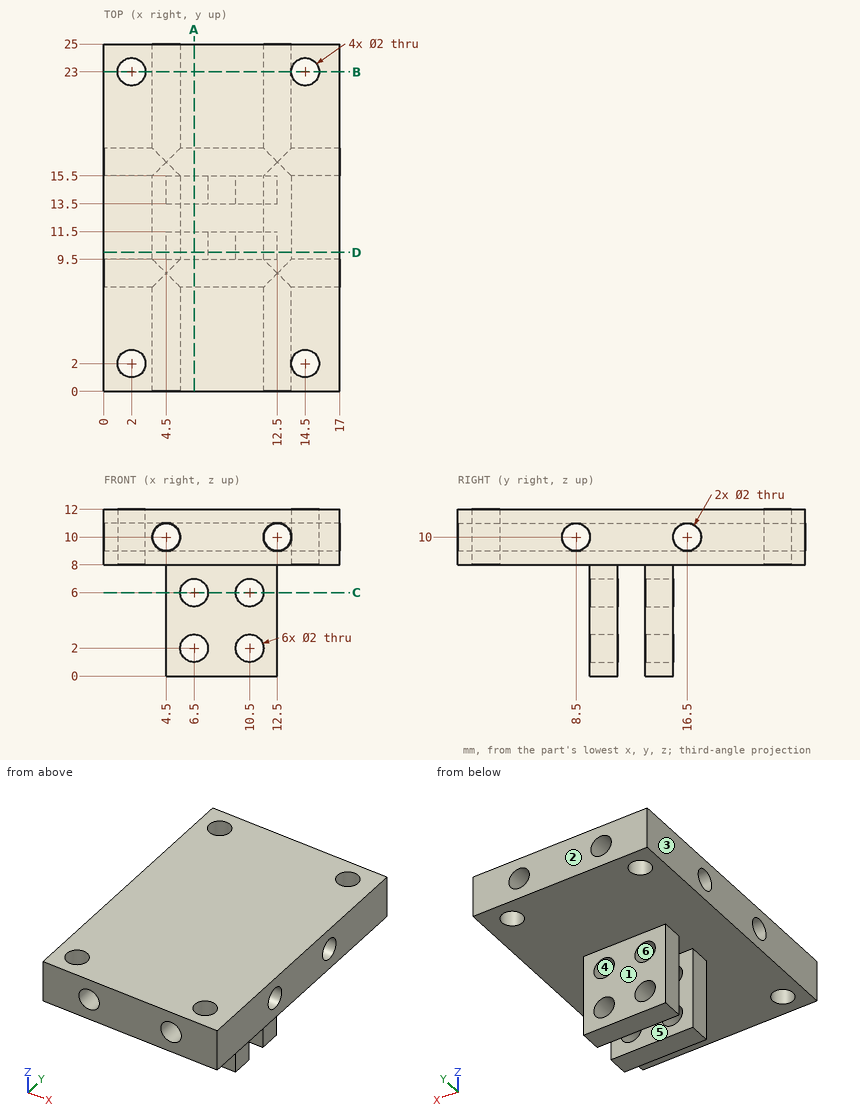
Could you check a few things on this drawing? It's one solid part, dimensions in mm from its lowest x, y, z. A direction names the side the tool comes from. Coordinates: 2 decimals unless noted, no trailing zeros. Order: outer loops, then holes, each group sorted by start corner. A loop starts at its lowest first (then second) coordinate and runs counter-clockwise, first axis right, second up. Notation, with made-up numbers: M 79,49 L 130,49 A30 ccw 130,84 Z; hole C 12.5,29 d2. An arc over 180 degrees is marked long. Answer as a JSON object with one key per item and string values. Group by question number.
(1) Which directions (+Z, -Z, +X, -X, +Y, -Y) give clear straight access to the entire face, cutting with the end or side of a thin tool? Please do the marked faces 1 and 2.
(2) For pin 1 (2.5 mm diameter, centred on x = 10, z = 4.5, fed in from +Y); pin 2 (1.2 mm diameter, centred on x = 12.5, z = 10, fed in from +Y); pin 3 (2 mm diameter, centred on y = 14.5, z = 5, fed in from +X); pin 4 (3 mm diameter, centred on x = 4, y = 20.5, fed in from -Z), each with a flat end and sliding along its axis, tell me the tip position at first contact or that it passes through.
(3) I need wall thicknesses on probe 1 along Z at (x, y) = (10.5, 14.1); probe 2 along X at (y, z) = (11.5, 10); probe 3 along Y at (x, z) = (10.25, 10). Which ranges of each line are inside material? Lowest first, please.
(4) Suppose I cut it at C-C, the plane z = 6. Please give me the cut outline in (x, y), then the cut area to 3 significant figures.
(5) Suppose I cut it at B-B, the plane y = 23. Please give me the cut outline in (x, z).
(6) If we mould it in two halves opening along X, with no side actions, what happens to the marked faces 3, 4, 5 and 6? For each: released by +X, released by -X, zero draft, split by the parting line, or undercut.
(7) Suppose I cut it at D-D, the plane y = 10. Please give me the cut outline in (x, z), then the cut area to 3 significant figures.
(8) Suppose I cut it at A-A, the plane x = 6.5. State how many separate pieces and enclosed holes the cut face has, then the cut area to 3 significant figures.
Values found:
{
 "1": {"face 1": "-Z, +X, -X, +Y", "face 2": "+Z, -Z, +X, -X, +Y"},
 "2": {"pin 1": "stops at y = 15.5", "pin 2": "passes through", "pin 3": "stops at x = 12.5", "pin 4": "stops at z = 8"},
 "3": {"probe 1": "z = 0 to 1, 3 to 5, 7 to 12", "probe 2": "x = 0 to 3.5, 5.5 to 11.5, 13.5 to 17", "probe 3": "y = 0 to 7.5, 9.5 to 15.5, 17.5 to 25"},
 "4": {"outline": "M 4.5,9.5 L 5.5,9.5 L 5.5,11.5 L 4.5,11.5 Z; M 4.5,13.5 L 5.5,13.5 L 5.5,15.5 L 4.5,15.5 Z; M 7.5,9.5 L 9.5,9.5 L 9.5,11.5 L 7.5,11.5 Z; M 7.5,13.5 L 9.5,13.5 L 9.5,15.5 L 7.5,15.5 Z; M 11.5,9.5 L 12.5,9.5 L 12.5,11.5 L 11.5,11.5 Z; M 11.5,13.5 L 12.5,13.5 L 12.5,15.5 L 11.5,15.5 Z", "area": "16.0 mm^2"},
 "5": {"outline": "M 0,8 L 1,8 L 1,12 L 0,12 Z; M 3,8 L 13.5,8 L 13.5,12 L 3,12 Z; M 15.5,8 L 17,8 L 17,12 L 15.5,12 Z; hole C 4.5,10 d2; hole C 12.5,10 d2"},
 "6": {"face 3": "released by -X", "face 4": "undercut", "face 5": "zero draft", "face 6": "undercut"},
 "7": {"outline": "M 0,8 L 4.5,8 L 4.5,0 L 12.5,0 L 12.5,8 L 17,8 L 17,12 L 0,12 Z; hole C 4.5,10 d2; hole C 6.5,2 d2; hole C 6.5,6 d2; hole C 10.5,2 d2; hole C 10.5,6 d2; hole C 12.5,10 d2", "area": "113 mm^2"},
 "8": {"separate pieces": "5", "enclosed holes": "2", "area": "110 mm^2"}
}
